Autodesk Inventor part; units mm, degrees
ref_plane "YZ Plane" through (0, 0, 0) normal (1, 0, 0) x (0, 1, 0)
ref_plane "XZ Plane" through (0, 0, 0) normal (0, 1, 0) x (-1, 0, 0)
ref_plane "XY Plane" through (0, 0, 0) normal (0, 0, 1) x (1, 0, 0)
sketch "Sketch1" plane through (0, 0, 0) normal (0, 0, 1) x (1, 0, 0)
  line L0 (0, 0) -> (25.4, 0)
  line L1 (25.4, 0) -> (25.4, -12.7)
  line L2 (25.4, -12.7) -> (0, -12.7)
  line L3 (0, -12.7) -> (0, 0)
  dimension "d0" = 25.4
  dimension "d1" = 12.7
extrude "Extrusion1" add sketch "Sketch1" along normal blind 3.175
hole "Hole1" at (2.933, -3.2804, 3.175) direction (0, 0, -1) diameter 3.175 depth 3.175 tip angle 118
fillet "Fillet1" radius 3.175 4 edges at (25.4, 0, 1.5875) (0, 0, 1.5875) (0, -12.7, 1.5875) (25.4, -12.7, 1.5875)
properties part number "Keychain_Bowen"
The listing builds one solid part. Answer for the finished solid, in the listing's coordinates (mm). Give positions to 0.01 mm unless a question says otherwise; leave off trailing zeros. Order: outer loops, then holes, each group sorted by start corner. A loop starts at its lowest first (then second) coordinate and runs counter-clockwise, first axis right, second up. Notation, with made-up numbers: (77.25, -22.75) -> (123.25, -22.75) arc R23 cw to (123.25, -9.75) -> close; hole circle Ø3 at (37.25, 21.25). An arc over 180 degrees is marked (long way). Answer as a JSON object with one key per item and string values. Group by question number.
Item 1: Determine the mould class of faces 1 (the cylindrical face through (1.36, -3.07, 1.57)), 2 (the flat face through (13, -6, 3.175)), 3 (the cylindrical face through (24.45, -11.79, 1.61)) for opening direction X: pulls with the +X half, pulls with the -X half, needs draft (parallel to the pull), parting line crosses it, or undercut.
Item 2: Consider L1, parallel to X at y = -3.25, z = 2.4; L2, parallel to X at y = -4.25, z = 1.6; L3, parallel to Y at x = 4, z = 1.25. Determine where each line is inside the solid, lowest interval first. Write a range as from..to.
Item 3: The part is cut by section B-B on y = -2. Write down the section's boundary in (x, z) (3 decimals).
Item 4: The part is cut by section D-D on y = -11. Write down the section's boundary in (x, z) (3 decimals).
Item 5: The part is cut by section C-C on x = 23.5. Write down the section's boundary in (y, z) (3 decimals).
Result set:
{
 "1": {"face 1": "undercut", "face 2": "needs draft", "face 3": "pulls with the +X half"},
 "2": {"L1": "0..1.35, 4.52..25.4", "L2": "0..1.68, 4.19..25.4", "L3": "-12.7..-4.46, -2.1..0"},
 "3": {"outline": "(0.225, 0) -> (1.995, 0) -> (1.995, 3.175) -> (0.225, 3.175) -> close; (3.871, 0) -> (25.175, 0) -> (25.175, 3.175) -> (3.871, 3.175) -> close"},
 "4": {"outline": "(0.363, 0) -> (25.037, 0) -> (25.037, 3.175) -> (0.363, 3.175) -> close"},
 "5": {"outline": "(-12.433, 0) -> (-0.267, 0) -> (-0.267, 3.175) -> (-12.433, 3.175) -> close"}
}
